Geometry check sheet. Reference: the model listing, model coordinates, mm. A direction names the side the tool comes from. Round coordinates to 2 decimals unless told otherwise and drop trailing zeros. Order: outer loops, then holes, each group sorted by start corner. A loop starts at its lowest first (then second) coordinate and runs counter-clockwise, first axis right, second up. Notation, with made-up numbers: (81, 23.25) -> (116, 23.25) arc R18 ccw to (116, 50.25) -> close; hole circle Ø3 at (22, -19.75). An arc over 180 degrees is marked (long way). Answer as a JSON object with one key per item and string values. Group by question number.
from build123d import *

# Parameters (mm, degrees)
RECTANGLEBOX_DEPTH      = 2
RECTANGLEBOX_DEPTH_BACK = 10
SKETCHREC_W             = 200
SKETCHREC_H             = 70
RECTANGLER_R            = 2
RECTANGLEC_START        = -98
RECTANGLEC_OUTLINE_W    = 10
RECTANGLEC_OUTLINE_H    = 66
RECTANGLEC_DEPTH        = 196


# Read off the part's stored shape, not the designer's step: RectangleC
with BuildPart() as part:
    # SketchRec → RectangleBox (new, two sides: drawn at the far end of the back side and taken through both)
    with BuildSketch(Plane(origin=(0, 0, 0), x_dir=(1, 0, 0), z_dir=(0, 1, 0)).offset(-RECTANGLEBOX_DEPTH_BACK)):
        Rectangle(SKETCHREC_W, SKETCHREC_H)
    extrude(amount=RECTANGLEBOX_DEPTH + RECTANGLEBOX_DEPTH_BACK)

    # RectangleR
    rectangler_edges = [part.edges().sort_by_distance(p)[0] for p in [
        (100, 2, 0),
        (0, 2, -35),
        (-100, 2, 0),
        (0, 2, 35),
        (100, -4, 35),
        (-100, -4, 35),
        (-100, -4, -35),
        (100, -4, -35),
    ]]
    fillet(rectangler_edges, radius=RECTANGLER_R)

    # RectangleC outline → RectangleC (cut)
    with BuildSketch(Plane.YZ.offset(RECTANGLEC_START)):
        with Locations((-5, 0)):
            Rectangle(RECTANGLEC_OUTLINE_W, RECTANGLEC_OUTLINE_H)
    extrude(amount=RECTANGLEC_DEPTH, mode=Mode.SUBTRACT)


solid = part.part
Item 1: Sectioned sample at C-C, the plane z = -8.5. Enter the section's corners in (x, y), then the cut area to 3 significant figures.
Item 2: Thickness scan on L1, parallel to X at y = -4.5, z = -10; L2, parallel to Z at x = 20, y = -1.5; L3, parallel to Y at x = -69.5, z = 17.5. Record the ranges inside material, lowest first.
Item 3: Sectioned sample at A-A, the plane y = -4.5. Enter the section's corners in (x, z).
Item 4: Mould release check, pull along Z, two halves, no side actions. Record for faces 1 (the flat face through (-1, -5, -35)), 2 (the flat face through (-1, 2, 0)), 3 (the flat face through (-1, -5, 33)): pulls with the +Z half, pulls with the -Z half, needs draft (parallel to the pull), parting line crosses it, or undercut.
Item 5: Set-up check for faces 4 (the flat face through (98, -5, 0)), 5 (the flat face through (0, -10, -34)): record each of +Z, -Z, +X, -X, +Y, -Y from which the full face is reachable in a straight line by a thin tool's end or side.
Item 6: Sectioned sample at B-B, the plane x = 22.5. Enter the section's corners in (y, z), then the cut area to 3 significant figures.
Result:
{
 "1": {"outline": "(-100, -10) -> (-98, -10) -> (-98, 0) -> (98, 0) -> (98, -10) -> (100, -10) -> (100, 0) arc R2 ccw to (98, 2) -> (-98, 2) arc R2 ccw to (-100, 0) -> close", "area": "438 mm2"},
 "2": {"L1": "x = -100 to -98, 98 to 100", "L2": "z = -35 to -33, 33 to 35", "L3": "y = 0 to 2"},
 "3": {"outline": "(-100, -33) arc R2 ccw to (-98, -35) -> (98, -35) arc R2 ccw to (100, -33) -> (100, 33) arc R2 ccw to (98, 35) -> (-98, 35) arc R2 ccw to (-100, 33) -> close; hole (-98, -33) -> (98, -33) -> (98, 33) -> (-98, 33) -> close"},
 "4": {"face 1": "pulls with the -Z half", "face 2": "needs draft", "face 3": "undercut"},
 "5": {"face 4": "-Y", "face 5": "+Z, -Z, +X, -X, -Y"},
 "6": {"outline": "(-10, -35) -> (0, -35) arc R2 ccw to (2, -33) -> (2, 33) arc R2 ccw to (0, 35) -> (-10, 35) -> (-10, 33) -> (0, 33) -> (0, -33) -> (-10, -33) -> close", "area": "178 mm2"}
}
